Work out the finished part from the listing and answer in its coordinate system (mm). A direction names the side the tool comes from. Round coordinates to 2 decimals unless told otherwise and drop trailing zeros. Write each loop counter-clockwise with the first axis right and the second up, starting at its lowest first coordinate (ties: lowest second). Pieces come first, ordered by that corner, then holes. Notation, with made-up numbers: (49.25, 42.5) -> (63.25, 42.5) arc R21 cw to (63.25, 49.5) -> close; hole circle Ø6 at (79.5, -9). An arc over 180 degrees is marked (long way). One line per question, with ' | ' between items. Start each with the question number.
```python
from build123d import *

# Parameters (mm, degrees)
F0_W     = 150
F0_H     = 150
F1_DEPTH = 9
F2_W     = 150
F2_H     = 150
F2_W_2   = 132
F2_H_2   = 132
F3_DEPTH = 141
F4_R     = 20.5
F5_DEPTH = 9
F6_R     = 35
F7_DEPTH = 9
F9_DEPTH = 9


with BuildPart() as f1:
    # F0 (on Front) → F1 (new body)
    with BuildSketch(Plane.XZ):
        Rectangle(F0_W, F0_H)
    extrude(amount=F1_DEPTH)

    # F2 (on face) → F3 (join)
    with BuildSketch(Plane.XZ.offset(9)):
        Rectangle(F2_W, F2_H)
        Rectangle(F2_W_2, F2_H_2, mode=Mode.SUBTRACT)
    extrude(amount=F3_DEPTH)

    # F4 (on face) → F5 (cut, through all)
    with BuildSketch(Plane(origin=(0, 0, -75), x_dir=(1, 0, 0), z_dir=(0, 0, -1))):
        with Locations((0, 75)):
            Circle(F4_R)
    extrude(amount=-F5_DEPTH, mode=Mode.SUBTRACT)

    # F6 (on face) → F7 (cut, through all)
    with BuildSketch(Plane(origin=(0, 0, 0), x_dir=(-1, 0, 0), z_dir=(0, 1, 0))):
        Circle(F6_R)
    extrude(amount=-F7_DEPTH, mode=Mode.SUBTRACT)

    # F8 (on face) → F9 (cut, through all)
    with BuildSketch(Plane(origin=(0, 0, -75), x_dir=(1, 0, 0), z_dir=(0, 0, -1))):
        with BuildLine():
            ThreePointArc((55, 110), (63.698903, 109.948769), (65, 118.549972))
            ThreePointArc((65, 118.549972), (0, 136), (-65, 118.549972))
            ThreePointArc((-65, 118.549972), (-65.902612, 107.371324), (-55, 110))
            ThreePointArc((-55, 110), (0, 122.300128), (55, 110))
        make_face()
    extrude(amount=-F9_DEPTH, mode=Mode.SUBTRACT)


solid = f1.part
```
(1) A cutting plane is placed at B-B, the plane z = 0. Determine the outline of the cut face in (x, y).
(2) For faces 1 (the cylindrical face through (18.937, -67.148, -70.563)), 2 (the flat face through (-1, -74, 75)), 3 (the flat face through (66, -79, -1)), determine the directions among +Z, -Z, +X, -X, +Y, -Y from which every point of the face is accessible in a straight line to the end or side of a thin tool.
(3) Consider L1, parallel to Y at x = 0, z = -72; L2, parallel to X at y = -75.5, z = 39. Determine where each line is inside the solid, lowest interval first.
(4) A cutting plane is placed at A-A, the plane x = 0. Determine the outline of the cut face in (y, z), then the cut area to 3 significant figures.
(5) The mould has two halves that part along Z. Classify faces 4 (the flat face through (-66, -79, -1)), 5 (the cylindrical face through (63.597, -109.864, -70.563)), 6 (the flat face through (16, -57, -75)): +Z half, -Z half, draft (parallel to the pull), parting line (faces both ways), or undercut.
(6) Given pin 1 Ø3 at (x, z) = (-46.5, 13.5) entering from -Y; pin 2 Ø1.9 at (x, y) = (-67, -111.5) entering from -Z, each flat-ended and moving along its own axis, determine where each tip first touches the part or whether it passes through.
(7) A cutting plane is placed at D-D, the plane y = -19. Determine the outline of the cut face in (x, z).
(8) A cutting plane is placed at C-C, the plane y = -75. Determine the outline of the cut face in (x, z).
Returned:
1) outline: (-75, -150) -> (-66, -150) -> (-66, -9) -> (-35, -9) -> (-35, 0) -> (-75, 0) -> close; (35, -9) -> (66, -9) -> (66, -150) -> (75, -150) -> (75, 0) -> (35, 0) -> close
2) face 1: -Z | face 2: +Z, +X, -X, +Y, -Y | face 3: -Y
3) L1: -150 to -136, -122.3 to -95.5, -54.5 to 0 | L2: -75 to -66, 66 to 75
4) outline: (-150, -75) -> (-136, -75) -> (-136, -66) -> (-150, -66) -> close; (-150, 66) -> (-9, 66) -> (-9, 35) -> (0, 35) -> (0, 75) -> (-150, 75) -> close; (-122.3, -75) -> (-95.5, -75) -> (-95.5, -66) -> (-122.3, -66) -> close; (-54.5, -75) -> (0, -75) -> (0, -35) -> (-9, -35) -> (-9, -66) -> (-54.5, -66) -> close | area: 2,770 mm2
5) face 4: undercut | face 5: draft | face 6: -Z half
6) pin 1: y = -9 | pin 2: z = -66
7) outline: (-75, -75) -> (75, -75) -> (75, 75) -> (-75, 75) -> close; hole (-66, -66) -> (66, -66) -> (66, 66) -> (-66, 66) -> close
8) outline: (-75, -75) -> (-20.5, -75) -> (-20.5, -66) -> (-66, -66) -> (-66, 66) -> (66, 66) -> (66, -66) -> (20.5, -66) -> (20.5, -75) -> (75, -75) -> (75, 75) -> (-75, 75) -> close
